The listing builds one solid part. Answer for the finished solid, in the listing's coordinates (mm). Face numbers are marked on the shaded views. A direction names the side the tool comes from. Give positions to 0.01 mm unless a question says otherwise; leave off trailing zeros. Write each loop counter-clockwise with the first axis right and the second up, starting at its lowest first coordinate (ties: lowest second). Pieces come first, ordered by that corner, then holes. Notation, with made-up numbers: (-34, 12.5) -> (-26, 12.5) arc R32 ccw to (-26, 41.5) -> close; hole circle Ø2 at (69.25, 26). An arc over 180 degrees is marked (long way). One line per question, with ' | ' between items.
Autodesk Inventor part; units mm, degrees
ref_plane "YZ Plane" through (0, 0, 0) normal (1, 0, 0) x (0, 1, 0)
ref_plane "XZ Plane" through (0, 0, 0) normal (0, 1, 0) x (-1, 0, 0)
ref_plane "XY Plane" through (0, 0, 0) normal (0, 0, 1) x (1, 0, 0)
sketch "Sketch1" plane through (0, 0, 0) normal (0, 0, 1) x (1, 0, 0)
  arc A0 (-17.1176, 3.6385) -> (-17.1176, -3.6385) centre (0, 0) ccw
  circle A1 centre (0, 0) radius 7.5
  arc A2 (-15.4058, 3.2746) -> (-15.4058, -3.2746) centre (0, 0) ccw
  circle A3 centre (0, 0) radius 9.25
  line L0 (0, 0) -> (-17.5, 0) construction
  line L1 (-15.7182, -1) -> (-9.1958, -1)
  line L2 (-15.7182, 1) -> (-9.1958, 1)
  line L3 (-15.4058, 3.2746) -> (-17.1176, 3.6385)
  line L4 (-15.4058, -3.2746) -> (-17.1176, -3.6385)
  line L5 (0, 0) -> (-17.1176, 3.6385) construction
  arc A4 (-16.6435, -5.4078) -> (-13.005, -11.7098) centre (0, 0) ccw
  arc A5 (-14.9791, -4.867) -> (-11.7045, -10.5388) centre (0, 0) ccw
  line L6 (-13.1124, -8.7251) -> (-7.4638, -5.4639)
  line L7 (-14.1124, -6.9931) -> (-8.4638, -3.7319)
  line L8 (-14.9791, -4.867) -> (-16.6435, -5.4078)
  line L9 (-11.7045, -10.5388) -> (-13.005, -11.7098)
  arc A6 (-11.7098, -13.005) -> (-5.4078, -16.6435) centre (0, 0) ccw
  arc A7 (-10.5388, -11.7045) -> (-4.867, -14.9791) centre (0, 0) ccw
  line L10 (-6.9931, -14.1124) -> (-3.7319, -8.4638)
  line L11 (-8.7251, -13.1124) -> (-5.4639, -7.4638)
  line L12 (-10.5388, -11.7045) -> (-11.7098, -13.005)
  line L13 (-4.867, -14.9791) -> (-5.4078, -16.6435)
  arc A8 (-3.6385, -17.1176) -> (3.6385, -17.1176) centre (0, 0) ccw
  arc A9 (-3.2746, -15.4058) -> (3.2746, -15.4058) centre (0, 0) ccw
  line L14 (1, -15.7182) -> (1, -9.1958)
  line L15 (-1, -15.7182) -> (-1, -9.1958)
  line L16 (-3.2746, -15.4058) -> (-3.6385, -17.1176)
  line L17 (3.2746, -15.4058) -> (3.6385, -17.1176)
  arc A10 (5.4078, -16.6435) -> (11.7098, -13.005) centre (0, 0) ccw
  arc A11 (4.867, -14.9791) -> (10.5388, -11.7045) centre (0, 0) ccw
  line L18 (8.7251, -13.1124) -> (5.4639, -7.4638)
  line L19 (6.9931, -14.1124) -> (3.7319, -8.4638)
  line L20 (4.867, -14.9791) -> (5.4078, -16.6435)
  line L21 (10.5388, -11.7045) -> (11.7098, -13.005)
  arc A12 (13.005, -11.7098) -> (16.6435, -5.4078) centre (0, 0) ccw
  arc A13 (11.7045, -10.5388) -> (14.9791, -4.867) centre (0, 0) ccw
  line L22 (14.1124, -6.9931) -> (8.4638, -3.7319)
  line L23 (13.1124, -8.7251) -> (7.4638, -5.4639)
  line L24 (11.7045, -10.5388) -> (13.005, -11.7098)
  line L25 (14.9791, -4.867) -> (16.6435, -5.4078)
  arc A14 (17.1176, -3.6385) -> (17.1176, 3.6385) centre (0, 0) ccw
  arc A15 (15.4058, -3.2746) -> (15.4058, 3.2746) centre (0, 0) ccw
  line L26 (15.7182, 1) -> (9.1958, 1)
  line L27 (15.7182, -1) -> (9.1958, -1)
  line L28 (15.4058, -3.2746) -> (17.1176, -3.6385)
  line L29 (15.4058, 3.2746) -> (17.1176, 3.6385)
  arc A16 (16.6435, 5.4078) -> (13.005, 11.7098) centre (0, 0) ccw
  arc A17 (14.9791, 4.867) -> (11.7045, 10.5388) centre (0, 0) ccw
  line L30 (13.1124, 8.7251) -> (7.4638, 5.4639)
  line L31 (14.1124, 6.9931) -> (8.4638, 3.7319)
  line L32 (14.9791, 4.867) -> (16.6435, 5.4078)
  line L33 (11.7045, 10.5388) -> (13.005, 11.7098)
  arc A18 (11.7098, 13.005) -> (5.4078, 16.6435) centre (0, 0) ccw
  arc A19 (10.5388, 11.7045) -> (4.867, 14.9791) centre (0, 0) ccw
  line L34 (6.9931, 14.1124) -> (3.7319, 8.4638)
  line L35 (8.7251, 13.1124) -> (5.4639, 7.4638)
  line L36 (10.5388, 11.7045) -> (11.7098, 13.005)
  line L37 (4.867, 14.9791) -> (5.4078, 16.6435)
  arc A20 (3.6385, 17.1176) -> (-3.6385, 17.1176) centre (0, 0) ccw
  arc A21 (3.2746, 15.4058) -> (-3.2746, 15.4058) centre (0, 0) ccw
  line L38 (-1, 15.7182) -> (-1, 9.1958)
  line L39 (1, 15.7182) -> (1, 9.1958)
  line L40 (3.2746, 15.4058) -> (3.6385, 17.1176)
  line L41 (-3.2746, 15.4058) -> (-3.6385, 17.1176)
  arc A22 (-5.4078, 16.6435) -> (-11.7098, 13.005) centre (0, 0) ccw
  arc A23 (-4.867, 14.9791) -> (-10.5388, 11.7045) centre (0, 0) ccw
  line L42 (-8.7251, 13.1124) -> (-5.4639, 7.4638)
  line L43 (-6.9931, 14.1124) -> (-3.7319, 8.4638)
  line L44 (-4.867, 14.9791) -> (-5.4078, 16.6435)
  line L45 (-10.5388, 11.7045) -> (-11.7098, 13.005)
  arc A24 (-13.005, 11.7098) -> (-16.6435, 5.4078) centre (0, 0) ccw
  arc A25 (-11.7045, 10.5388) -> (-14.9791, 4.867) centre (0, 0) ccw
  line L46 (-14.1124, 6.9931) -> (-8.4638, 3.7319)
  line L47 (-13.1124, 8.7251) -> (-7.4638, 5.4639)
  line L48 (-11.7045, 10.5388) -> (-13.005, 11.7098)
  line L49 (-14.9791, 4.867) -> (-16.6435, 5.4078)
  point P0 (-15.1554, -8.75)
  point P1 (-8.75, -15.1554)
  point P2 (0, -17.5)
  point P3 (8.75, -15.1554)
  point P4 (15.1554, -8.75)
  point P5 (17.5, 0)
  point P6 (15.1554, 8.75)
  point P7 (8.75, 15.1554)
  point P8 (0, 17.5)
  point P9 (-8.75, 15.1554)
  point P10 (-15.1554, 8.75)
  dimension "d0" = 35
  dimension "d1" = 15
  dimension "d2" = 1.75
  dimension "d3" = 1.75
  dimension "d6" = 1
  dimension "d7" = 12
  dimension "d10" = 360
extrude "Extrusion1" add sketch "Sketch1" along normal blind 16
properties part number "STATOR"
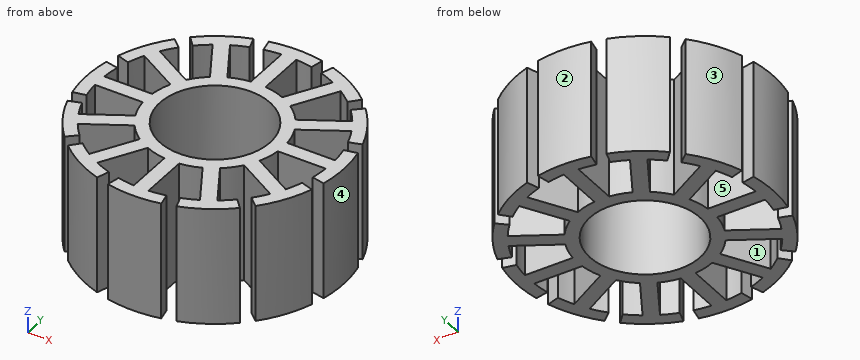
Item 1: Find section C-C (y = -8). Write down the section's boundary in (x, z).
Answers below:
outline: (-15.56, 0) -> (-11.86, 0) -> (-11.86, 16) -> (-15.56, 16) -> close; (-5.77, 0) -> (5.77, 0) -> (5.77, 16) -> (-5.77, 16) -> close; (11.86, 0) -> (15.56, 0) -> (15.56, 16) -> (11.86, 16) -> close
Item 2: Consider line 1 (Y direction, x = 1.5, z = 12.25); line 2 (X direction, y = -6, z = 11.75); line 3 (Y direction, x = -9.5, z = 4.5). Determine where each line is inside the solid, lowest interval first. Write a range as [from, to].
Answers below:
line 1: [-17.44, -15.68], [-9.13, -7.35], [7.35, 9.13], [15.68, 17.44] | line 2: [-16.44, -14.56], [-12.39, -8.39], [-7.04, -4.5], [4.5, 7.04], [8.39, 12.39], [14.56, 16.44] | line 3: [-14.7, -12.56], [-6.64, -4.33], [-1, 1], [4.33, 6.64], [12.56, 14.7]
Item 3: Find section A-A (x = 0). Write down the section's boundary in (y, z).
Answers below:
outline: (-17.5, 0) -> (-7.5, 0) -> (-7.5, 16) -> (-17.5, 16) -> close; (7.5, 0) -> (17.5, 0) -> (17.5, 16) -> (7.5, 16) -> close
Item 4: Flat-ended cylindrical pins translate along their axes: pin 1 (5 mm diameter, centred on y = 12.5, z = 11, fed in from +X); pin 2 (7 mm diameter, centred on x = 12, z = 7, fed in from +Y); pin 3 (5 mm diameter, centred on y = -13, z = 4.5, fed in from -X). Find the tip coordinate at first contact, or state that the pin passes through.
Answers below:
pin 1: x = 14.36 | pin 2: y = 15.3 | pin 3: x = -14
Item 5: Determine the mould class of the marked faces 1, 2 and 3 for opening direction X: pulls with the +X half, pulls with the -X half, needs draft (parallel to the pull), parting line crosses it, or undercut.
Answers below:
face 1: undercut | face 2: parting line crosses it | face 3: pulls with the -X half
Item 6: A tool of negligible diameter and unlimited length cuts with its end or side. For the marked faces 4 and 5, from which of +Z, -Z, +X, -X, +Y, -Y can it reach the whole face along a straight path? Write none if from no direction.
Answers below:
face 4: +Z, -Z, +X | face 5: +Z, -Z
